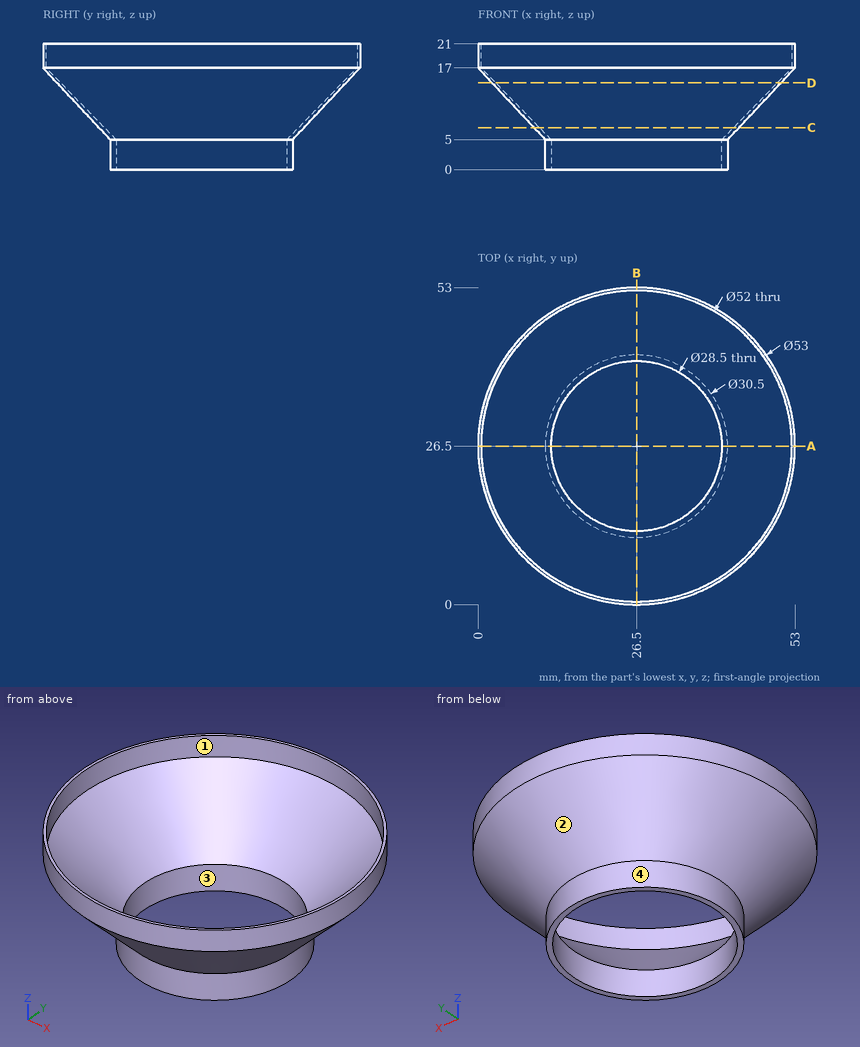
The figure shows three views and two pictorial views of one solid part (mm, origin at its lowest corner). Answer the questions. A direction names the side the tool comes from. Give positions to 0.01 mm unless a question says otherwise; leave off trailing zeros. Write each loop counter-clockwise with the first axis right and the second up, starting at its lowest first coordinate (ties: lowest second). Pieces come first, ordered by that corner, then holes. Notation, with made-up numbers: (-9, 80.5) - (18, 80.5) arc R12 ccw to (18, 91.5) - close; hole circle Ø7 at (80, -2.75). An arc over 180 degrees is marked (long way). Use CSV: the item, a comma, the result in double quotes. Start each with the question number.
Item 1: The part is cut by section D-D, the plane z = 14.5. Give the vertices of the cut face in (x, y).
Item 2: Consider line 1 (X direction, y = 26.5, z = 19.8); line 2 (Y direction, x = 26.5, z = 1.45). Determine where each line is inside the solid, lowest interval first.
Item 3: Flat-ended cylindrical pins translate along their axes: P1, Ø5, axis at x = 13, z = 18, coming from the -Y side; P2, Ø2, axis at x = 26, z = 19, coming from the -Y side; P3, Ø2, axis at x = 9, y = 13, coming from the +Z side. Find the tip coordinate at first contact, or state that the pin passes through.
Item 4: For the marked faces 1 and 2, determine the directions among +Z, -Z, +X, -X, +Y, -Y from which every point of the face is accessible in a straight line to the end or side of a thin tool.
Item 5: The part is cut by section C-C, the plane z = 7. Give the vertices of the cut face in (x, y) (3 decimals).
Item 6: The part is cut by section A-A, the plane y = 26.5. Give the vertices of the cut face in (x, z), and give its area (3 significant figures).
Item 7: The mould has two halves that part along X. Classify the marked faces 3 and 4: pulls with the +X half, pulls with the -X half, needs draft (parallel to the pull), parting line crosses it, or undercut.
Taken from the geometry:
1,outline,"circle Ø48.31 at (26.5, 26.5); hole circle Ø47.1 at (26.5, 26.5)"
2,line 1,"0 to 0.5, 52.5 to 53"
2,line 2,"11.25 to 12.25, 40.75 to 41.75"
3,P1,"y = 2.39"
3,P2,"y = 0"
3,P3,"z = 14.04"
4,face 1,"+Z"
4,face 2,"-Z"
5,outline,"circle Ø34.25 at (26.5, 26.5); hole circle Ø32.417 at (26.5, 26.5)"
6,outline,"(0, 17) - (11.25, 5) - (11.25, 0) - (12.25, 0) - (12.25, 5) - (0.5, 17) - (0.5, 21) - (0, 21) - close; (40.75, 0) - (41.75, 0) - (41.75, 5) - (53, 17) - (53, 21) - (52.5, 21) - (52.5, 17) - (40.75, 5) - close"
6,area,"32.0 mm2"
7,face 3,"undercut"
7,face 4,"parting line crosses it"
